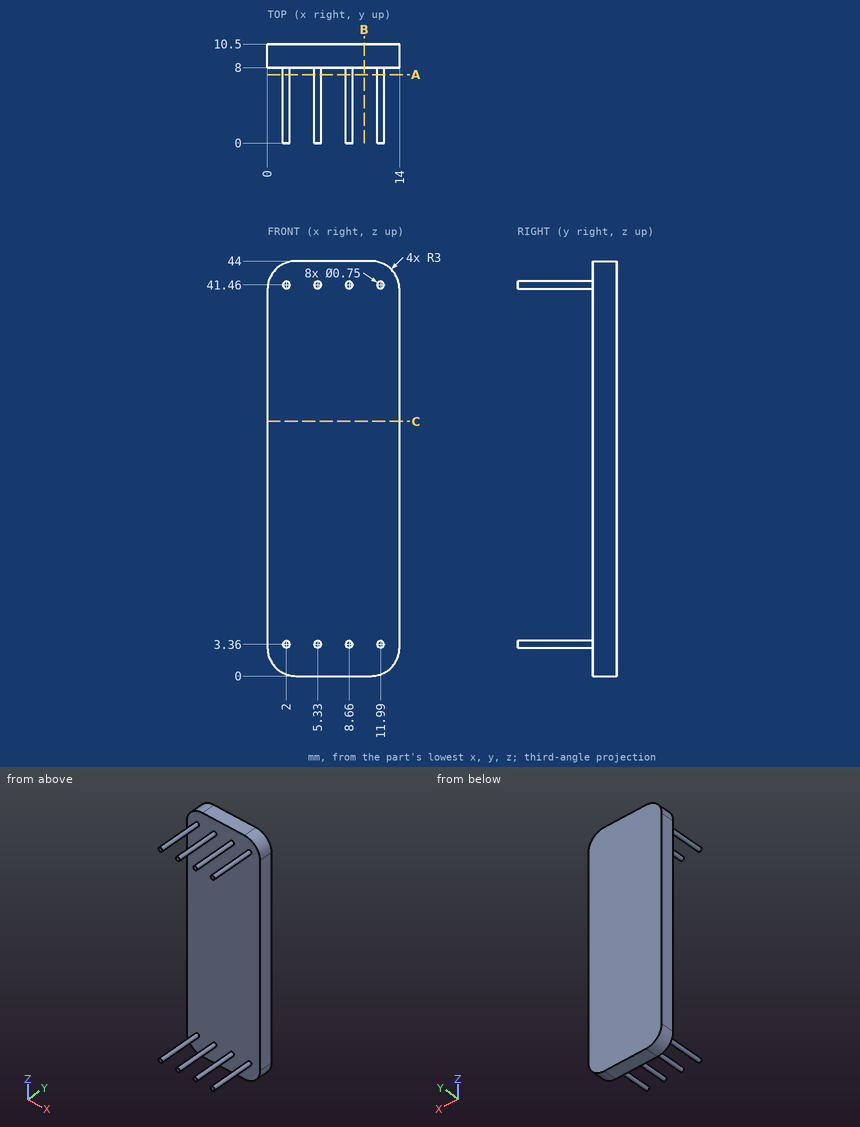
Drawing for the job (mm, zero at the part's lowest x, y, z). Round coordinates to 2 decimals unless told otherwise and drop trailing zeros. Order: outer loops, then holes, each group sorted by start corner. A loop starts at its lowest first (then second) coordinate and runs counter-clockwise, first axis right, second up. Notation, with made-up numbers: (42, 89) -> (68, 89) arc R25 ccw to (68, 113) -> close; hole circle Ø7 at (76, 45.5). An arc over 180 degrees is marked (long way). Write item = value, one per line. Start each with the question number.
(1) Cut at B-B, the plane x = 10.25. List the corners of the cut face in (y, z), then the cut area to 3 significant figures.
(2) Pin check, flat tips, straight feed: P1, Ø7, axis at x = 7, z = 26.5, coming from the -Y side; P2, Ø4, axis at x = 9.5, y = 4, coming from the -Z side (3 decimals); P3, Ø6, axis at y = 4.5, z = 36.5, coming from the -X side. Stop position of each tip, or through.
(3) Cut at A-A, the plane y = 7.25. List the corners of the cut face in (x, z) (3 decimals).
(4) Cut at C-C, the plane z = 27. List the corners of the cut face in (x, y).
(5) Probe line 1 (Z direction, x = 5.25, y = 2.75); line 2 (X direction, y = 6, z = 41.5); line 3 (Y direction, x = 1.25, z = 33.5). List the from-to ranges inside material, lowest first. Write a range as [from, to].
Model answer:
q1.outline = (8, 0) -> (10.5, 0) -> (10.5, 44) -> (8, 44) -> close
q1.area = 110 mm2
q2.P1 = 8
q2.P2 = 2.985
q2.P3 = through
q3.outline = circle Ø0.75 at (2, 3.36); circle Ø0.75 at (2, 41.46); circle Ø0.75 at (5.33, 3.36); circle Ø0.75 at (5.33, 41.46); circle Ø0.75 at (8.66, 3.36); circle Ø0.75 at (8.66, 41.46); circle Ø0.75 at (11.99, 3.36); circle Ø0.75 at (11.99, 41.46)
q4.outline = (0, 8) -> (14, 8) -> (14, 10.5) -> (0, 10.5) -> close
q5.line_1 = [2.99, 3.73], [41.09, 41.83]
q5.line_2 = [1.63, 2.37], [4.96, 5.7], [8.29, 9.03], [11.62, 12.36]
q5.line_3 = [8, 10.5]
